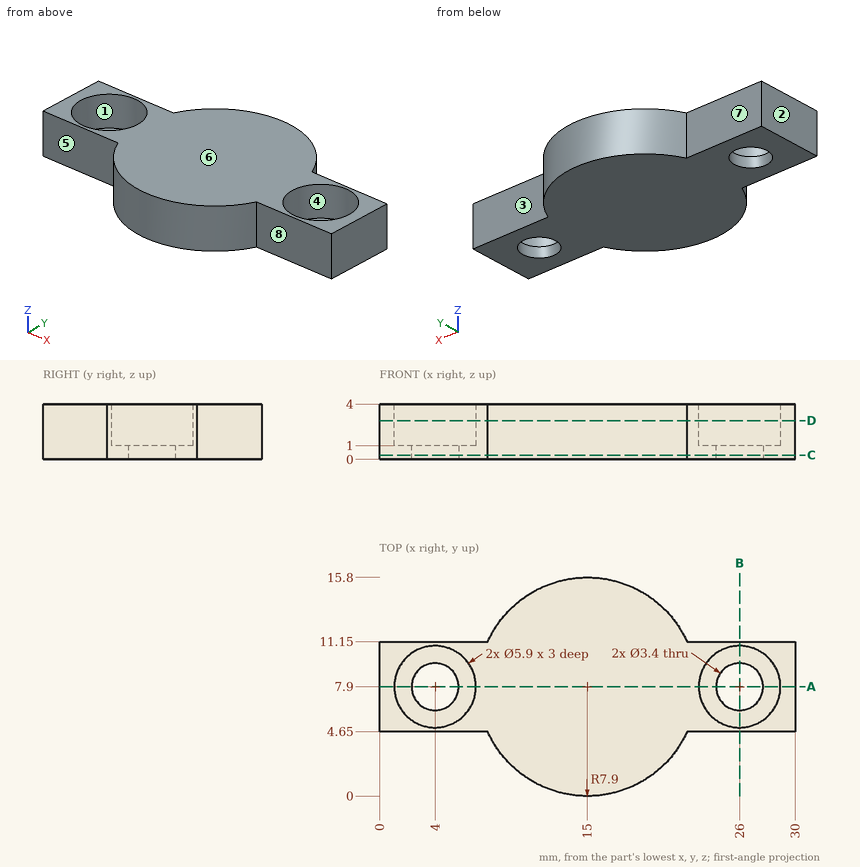
Check sheet for the drawn part. Datum: minimum x, y, z corner. Units: mm. A direction names the side the tool comes from. Round coordinates to 2 decimals unless told otherwise and drop trailing zeros. Loops run counter-clockwise (first coordinate to the right, second up) from the corner with the lowest first, then second, coordinate; pieces in that order, holes last. Notation, with made-up numbers: (42.5, -38.75) - (79.5, -38.75) arc R9 ccw to (79.5, -24.75) - close; hole circle Ø10 at (62.25, -10.5). An arc over 180 degrees is marked (long way). Answer as a JSON object with one key per item and string values. Group by question number.
Q1. Gauge pin test, flat end, axial feed: P1, Ø3, axis at x = 25, y = 8.5, coming from the +Z side. Record the tip position at first contact, or that the pin passes through.
Q2. Sectioned sample at B-B, the plane x = 26. Enter the section's corners in (y, z).
Q3. Set-up check for the marked faces 4, 5, 6, 7 and 8: record each of +Z, -Z, +X, -X, +Y, -Y from which the full face is reachable in a straight line by a thin tool's end or side.
Q4. Sectioned sample at C-C, the plane z = 0.3. Enter the section's corners in (x, y).
Q5. Sectioned sample at D-D, the plane z = 2.8. Enter the section's corners in (x, y), plus the area to 3 significant figures.
Q6. Mould release check, pull along X, two halves, no side actions. Record for the marked faces 1, 2 and 3: released by +X, released by -X, zero draft, split by the parting line, or undercut.
Q7. Scan lines: line 1 along X through (y, z) = (8, 2.3); line 2 along Y through (x, z) = (26, 1.8); line 3 along Y through (x, z) = (26, 0.5). Record each from-to range of solid material in increasing order. Write a range as [from, to].
Q8. Sectioned sample at A-A, the plane y = 7.9. Enter the section's corners in (x, z).
Solution:
{
 "1": {"P1": "stops at z = 1"},
 "2": {"outline": "(4.65, 0) - (6.2, 0) - (6.2, 1) - (4.95, 1) - (4.95, 4) - (4.65, 4) - close; (9.6, 0) - (11.15, 0) - (11.15, 4) - (10.85, 4) - (10.85, 1) - (9.6, 1) - close"},
 "3": {"face 4": "+Z", "face 5": "+Z, -Z, -X, -Y", "face 6": "+Z, +X, -X, +Y, -Y", "face 7": "+Z, -Z, -X, +Y", "face 8": "+Z, -Z, +X, -Y"},
 "4": {"outline": "(0, 4.65) - (7.8, 4.65) arc R7.9 ccw to (22.2, 4.65) - (30, 4.65) - (30, 11.15) - (22.2, 11.15) arc R7.9 ccw to (7.8, 11.15) - (0, 11.15) - close; hole circle Ø3.4 at (4, 7.9); hole circle Ø3.4 at (26, 7.9)"},
 "5": {"outline": "(0, 4.65) - (7.8, 4.65) arc R7.9 ccw to (22.2, 4.65) - (30, 4.65) - (30, 11.15) - (22.2, 11.15) arc R7.9 ccw to (7.8, 11.15) - (0, 11.15) - close; hole circle Ø5.9 at (4, 7.9); hole circle Ø5.9 at (26, 7.9)", "area": "237 mm²"},
 "6": {"face 1": "undercut", "face 2": "released by -X", "face 3": "zero draft"},
 "7": {"line 1": "x = [0, 1.05], [6.95, 23.05], [28.95, 30]", "line 2": "y = [4.65, 4.95], [10.85, 11.15]", "line 3": "y = [4.65, 6.2], [9.6, 11.15]"},
 "8": {"outline": "(0, 0) - (2.3, 0) - (2.3, 1) - (1.05, 1) - (1.05, 4) - (0, 4) - close; (5.7, 0) - (24.3, 0) - (24.3, 1) - (23.05, 1) - (23.05, 4) - (6.95, 4) - (6.95, 1) - (5.7, 1) - close; (27.7, 0) - (30, 0) - (30, 4) - (28.95, 4) - (28.95, 1) - (27.7, 1) - close"}
}
